Check sheet for the modelled part. Datum: model origin and axes. Units: mm. A direction names the side the tool comes from. Coordinates: 2 decimals unless noted, no trailing zeros. Loops run counter-clockwise (first coordinate to the right, second up) from the corner with the lowest first, then second, coordinate; pieces in that order, holes last. Notation, with made-up numbers: M 63,45 L 97,45 A19 cw 97,60 Z; hole C 29.25,89 d1. An arc over 180 degrees is marked long. Return JSON: item names as keys, results as strings.
from build123d import *

# Parameters (mm, degrees)
SALIENTE_EXTRUIR1_DEPTH = 10.1
CROQUIS7_R              = 2.05
CORTAR_EXTRUIR1_DEPTH   = 0.5
CROQUIS11_W             = 20
CROQUIS11_H             = 1.2
CORTAR_EXTRUIR4_DEPTH   = 49.847437401
SALIENTE_EXTRUIR4_START = -7.7
SALIENTE_EXTRUIR4_DEPTH = 7.7
CROQUIS13_R             = 2.5
CORTAR_EXTRUIR5_DEPTH   = 1.5
CROQUIS14_R             = 3
SALIENTE_EXTRUIR5_DEPTH = 25
SALIENTE_EXTRUIR5_TAPER = 3


with BuildPart() as part:
    # Croquis1 → Saliente-Extruir1 (new body)
    with BuildSketch(Plane(origin=(0, 0, 0), x_dir=(1, 0, 0), z_dir=(0, 1, 0))):
        with BuildLine():
            Line((-33.071856209, -5.003625594), (33.023928918, -5.003625594))
            Line((33.023928918, -5.003625594), (33.023928918, 4.996374406))
            Line((33.023928918, 4.996374406), (-32.976071082, 4.996374406))
            ThreePointArc((-32.976071082, 4.996374406), (-46.113327984, 0.121751049), (-33.071856209, -5.003625594))
        make_face()
    extrude(amount=SALIENTE_EXTRUIR1_DEPTH)

    # Croquis7 → Cortar-Extruir1 (cut)
    with BuildSketch(Plane(origin=(0, 10.1, 0), x_dir=(1, 0, 0), z_dir=(0, 1, 0))):
        with Locations(Location((-38.613672015, 0.049915499, 0), (0, 0, 270))):
            Circle(CROQUIS7_R)
    extrude(amount=-CORTAR_EXTRUIR1_DEPTH, mode=Mode.SUBTRACT)

    # Croquis11 → Cortar-Extruir4 (cut, through all)
    with BuildSketch(Plane.XY.offset(5.003625594)):
        with Locations((23.023928918, 9.5)):
            Rectangle(CROQUIS11_W, CROQUIS11_H)
        with Locations((23.023928918, 0.6)):
            Rectangle(CROQUIS11_W, CROQUIS11_H)
    extrude(amount=-CORTAR_EXTRUIR4_DEPTH, mode=Mode.SUBTRACT)

    # Croquis12 → Saliente-Extruir4 (add)
    with BuildSketch(Plane(origin=(0, 8.9, 0), x_dir=(1, 0, 0), z_dir=(0, 1, 0)).offset(SALIENTE_EXTRUIR4_START)):
        with BuildLine():
            Line((33.023928918, 4.996374406), (33.023928918, -5.003625594))
            ThreePointArc((33.023928918, -5.003625594), (35.299630193, -5.437603932), (37.334427549, -6.54519285))
            ThreePointArc((37.334427549, -6.54519285), (44.24999745, -5.462503991), (43.306208076, 1.473387001))
            ThreePointArc((43.306208076, 1.473387001), (38.445512688, 4.053392135), (33.023928918, 4.996374406))
        make_face()
    extrude(amount=SALIENTE_EXTRUIR4_DEPTH)

    # Croquis13 → Cortar-Extruir5 (cut)
    with BuildSketch(Plane(origin=(0, 8.9, 0), x_dir=(1, 0, 0), z_dir=(0, 1, 0))):
        with Locations(Location((40.239901123, -2.476013165, 0), (0, 0, 270))):
            Circle(CROQUIS13_R)
    cortar_extruir5 = extrude(amount=-CORTAR_EXTRUIR5_DEPTH, mode=Mode.SUBTRACT)

    # Croquis14 → Saliente-Extruir5 (add)
    with BuildSketch(Plane.XZ):
        with Locations((-38.613672015, -0.049915499)):
            Circle(CROQUIS14_R)
    extrude(amount=SALIENTE_EXTRUIR5_DEPTH, taper=SALIENTE_EXTRUIR5_TAPER)

    # Simetría1: Cortar-Extruir5 across plane
    add(cortar_extruir5.mirror(Plane.ZX.offset(5.05)), mode=Mode.SUBTRACT)


solid = part.part
1) Section check A-A on y = 5. Record the cut outline in (x, z).
Answers:
{"outline": "M -33.07,5 A7.5 ccw long -32.98,-5 L 33.02,-5 A17.5 ccw 43.31,-1.47 A5 ccw 37.33,6.55 A7.5 cw 33.02,5 Z"}
2) Draft check along X on faces 5 (the face through (29, 1.2, 0)), 6 (the face through (-40.615, 9.854, -0.494)), 7 (the face through (-39, 9.6, 0)), 8 (the face through (-36.456, -12.675, -0.945)). Enter one of: +X half, -X half, draft (parallel to the pull), parting line (faces both ways), or undercut.
Answers:
{"face 5": "draft", "face 6": "undercut", "face 7": "undercut", "face 8": "parting line"}
3) Section check C-C on x = 6.5. Record the cut outline in (y, z), then the cut area to 3 significant figures.
Answers:
{"outline": "M 0,-5 L 10.1,-5 L 10.1,5 L 0,5 Z", "area": "101 mm²"}
4) Section check D-D on y = -8. Record the cut outline in (x, z), then the cut area to 3 significant figures.
Answers:
{"outline": "C -38.61,-0.05 d5.16", "area": "20.9 mm²"}
5) Go/stop test with flat-tipped pins: pin 1 Ø0.6 at (y, z) = (9.5, -1) entering from +X; pin 2 Ø3 at (x, y) = (14.5, 6) entering from +Z; pin 3 Ø4 at (x, z) = (40.24, 2.48) entering from -Y. Record where each tip stops, or that it passes through.
Answers:
{"pin 1": "x = 13.02", "pin 2": "z = 5", "pin 3": "y = 2.7"}
6) Set-up check for faces 1 (the face through (29, 8.9, 0)), 2 (the face through (40, 2.7, 2)), 3 (the face through (35.269, 4.996, 5.427)), 4 (the face through (40, 7.4, 2)): record each of +Z, -Z, +X, -X, +Y, -Y from which the full face is reachable in a straight line by a thin tool's end or side.
Answers:
{"face 1": "+Z, -Z, +X, +Y", "face 2": "-Y", "face 3": "+Z, +Y, -Y", "face 4": "+Y"}
7) Scan lines: line 1 along Y through (x, z) = (-28.5, 1.5); line 2 along X through (y, z) = (-18, -1.25); line 3 along X through (y, z) = (2.5, 1). Record each from-to range of solid material in increasing order. Write a range as [from, to].
Answers:
{"line 1": "[0, 10.1]", "line 2": "[-40.28, -36.94]", "line 3": "[-46.04, 38.22], [42.26, 45.02]"}
8) Section check B-B on x = 29. Record the cut outline in (y, z), then the cut area to 3 significant figures.
Answers:
{"outline": "M 1.2,-5 L 8.9,-5 L 8.9,5 L 1.2,5 Z", "area": "77.0 mm²"}
